Autodesk Inventor part; units mm, degrees
ref_plane "YZ Plane" through (0, 0, 0) normal (1, 0, 0) x (0, 1, 0)
ref_plane "XZ Plane" through (0, 0, 0) normal (0, 1, 0) x (-1, 0, 0)
ref_plane "XY Plane" through (0, 0, 0) normal (0, 0, 1) x (1, 0, 0)
sketch "Sketch1" plane through (0, 0, 0) normal (0, 0, 1) x (1, 0, 0)
  circle A0 centre (0, 0) radius 1.75
  circle A1 centre (0, -5.8674) radius 1.75
  arc A2 (-3.175, -15.3924) -> (3.175, -15.3924) centre (0, -15.3924) ccw
  arc A3 (3.175, 0) -> (-3.175, 0) centre (0, 0) ccw
  line L0 (-3.175, 0) -> (-3.175, -15.3924)
  line L1 (3.175, 0) -> (3.175, -15.3924)
  dimension "d0" = 3.5
  dimension "d3" = 3.5
extrude "Extrusion1" add sketch "Sketch1" along normal blind 3.175
sketch "Sketch2" plane through (0, 0, 3.175) normal (0, 0, 1) x (1, 0, 0)
  arc A0 (-3.175, -15.3924) -> (3.175, -15.3924) centre (0, -15.3924) ccw
  arc A1 (-3.175, -21.7424) -> (3.175, -21.7424) centre (0, -21.7424) ccw
  line L0 (-3.175, 0) -> (-3.175, -15.3924)
  line L1 (-3.175, -21.7424) -> (-3.175, -15.3924)
  line L2 (3.175, -15.3924) -> (3.175, -21.7424)
  arc A2 (-3.175, -15.3924) -> (3.175, -15.3924) centre (0, -15.3924) ccw
  point P0 (0, 0)
  dimension "d10" = 6.35
extrude "Extrusion2" add sketch "Sketch2" against normal blind 3.175
sketch "Sketch7" plane through (0, 0, 3.175) normal (0, 0, 1) x (1, 0, 0)
  arc A0 (-3.175, -21.7424) -> (3.175, -21.7424) centre (0, -21.7424) ccw
  arc A1 (-3.175, -20.1549) -> (3.175, -20.1549) centre (0, -20.1549) ccw
  line L0 (3.175, -21.7424) -> (3.175, 0)
  line L1 (-3.175, 0) -> (-3.175, -21.7424)
  line L2 (-3.175, -21.7424) -> (-3.175, -20.1549)
  line L3 (3.175, -21.7424) -> (3.175, -20.1549)
  arc A2 (-3.175, -21.7424) -> (3.175, -21.7424) centre (0, -21.7424) ccw
  point P0 (0, 0)
extrude "Extrusion8" cut sketch "Sketch7" against normal blind 3.175
properties part number "Brake"
CAD build for the part. Positions are in the model's coordinates, mm. Round coordinates to 2 decimals unless told otherwise and drop trailing zeros. Order: outer loops, then holes, each group sorted by start corner. A loop starts at its lowest first (then second) coordinate and runs counter-clockwise, first axis right, second up. Notation, with made-up numbers: (78, 61) - (127, 61) arc R30 cw to (127, 98) - close; hole circle Ø2 at (42, -6). An arc over 180 degrees is marked (long way). Return JSON: item names as keys, results as strings.
(1) Cut at B-B (y = -0.5). Give the cut face in (x, z) (3 decimals), then the cut area to 3 significant figures.
Answer key:
{"outline": "(-3.175, 0) - (-1.677, 0) - (-1.677, 3.175) - (-3.175, 3.175) - close; (1.677, 0) - (3.175, 0) - (3.175, 3.175) - (1.677, 3.175) - close", "area": "9.51 mm^2"}
(2) Pull direction X, two halves, no side cores. Call faces 1 (the face through (1.617, 0.67, 1.565)), 2 (the face through (-3.175, -10, 2)), 3 (the face through (-0.07, 3.174, 1.565)): +X half, -X half, draft (parallel to the pull), parting line (faces both ways), or undercut.
Answer key:
{"face 1": "undercut", "face 2": "-X half", "face 3": "parting line"}
(3) Cut at D-D (x = 1). Give the cut face in (y, z) (3 decimals).
Answer key:
{"outline": "(-23.168, 0) - (-7.304, 0) - (-7.304, 3.175) - (-23.168, 3.175) - close; (-4.431, 0) - (-1.436, 0) - (-1.436, 3.175) - (-4.431, 3.175) - close; (1.436, 0) - (3.013, 0) - (3.013, 3.175) - (1.436, 3.175) - close"}
(4) Cut at C-C (z = 1.2). Give the cut face in (x, y) (3 decimals), then the cut area to 3 significant figures.
Answer key:
{"outline": "(-3.175, -20.155) arc R3.175 ccw to (3.175, -20.155) - (3.175, 0) arc R3.175 ccw to (-3.175, 0) - close; hole circle Ø3.5 at (0, -5.867); hole circle Ø3.5 at (0, 0)", "area": "140 mm^2"}
(5) Wall check: probe 1 along Y at (x, z) = (0, 1.6) (3 decimals); probe 2 along Y at (x, z) = (-1, 1.8); probe 3 along X at (y, z) = (0.5, 0.75). Give the ranges that are in metal, low to high. Write a range as from..to.
Answer key:
{"probe 1": "y = -23.33..-7.617, -4.117..-1.75, 1.75..3.175", "probe 2": "y = -23.17..-7.3, -4.43..-1.44, 1.44..3.01", "probe 3": "x = -3.14..-1.68, 1.68..3.14"}
(6) Cut at A-A (x = 0). Give the cut face in (y, z) (3 decimals), then the cut area to 3 significant figures.
Answer key:
{"outline": "(-23.33, 0) - (-7.617, 0) - (-7.617, 3.175) - (-23.33, 3.175) - close; (-4.117, 0) - (-1.75, 0) - (-1.75, 3.175) - (-4.117, 3.175) - close; (1.75, 0) - (3.175, 0) - (3.175, 3.175) - (1.75, 3.175) - close", "area": "61.9 mm^2"}
